Can you work these out from the model? Positions are in its coordinate system, mm. A direction names the side the tool comes from. Give positions to 0.01 mm unless a question says otherwise; leave off trailing zeros. Order: outer loops, then holes, each group sorted by start corner. A loop starts at its lowest first (then second) coordinate and runs counter-clockwise, first axis right, second up. Notation, with made-up numbers: M 44,-14 L 57,-14 A20 ccw 57,3 Z; hole C -36,-2 d3. An arc over 180 degrees is marked long. Write each question's results on one line, items separated by ' | '.
from build123d import *

# Parameters (mm, degrees)
BOSS_EXTRUDE1_DEPTH  = 3.6
CUT_EXTRUDE1_START   = 3.6
CUT_EXTRUDE1_DEPTH   = 1.6
SKETCH3_R            = 0.3
CUT_EXTRUDE2_DEPTH   = 78.737828629
BOSS_EXTRUDE3_DEPTH  = 3
BOSS_EXTRUDE3_TAPER  = 10
SKETCH3_2_R          = 0.3
CUT_EXTRUDE3_DEPTH   = 78.872780874
LPATTERN5_COUNT      = 7
LPATTERN5_PITCH      = 1.27
CHAMFER2_SIZE        = 0.2
FILLET2_R            = 1
BOSS_EXTRUDE4_DEPTH  = 26.2
SKETCH7_R            = 1.05
CUT_EXTRUDE4_DEPTH   = 82.036781772
SKETCH8_W            = 4
SKETCH8_H            = 5.4
CUT_EXTRUDE5_DEPTH   = 1.6
SKETCH9_R            = 1
CUT_EXTRUDE7_DEPTH   = 1
LPATTERN6_COUNT      = 5
LPATTERN6_PITCH      = 2.54
LPATTERN6_COUNT_DIR2 = 2
LPATTERN6_PITCH_DIR2 = 2.54
SKETCH10_R           = 1
CUT_EXTRUDE8_DEPTH   = 1
BOSS_EXTRUDE5_DEPTH  = 1
LPATTERN7_COUNT      = 3
LPATTERN7_PITCH      = 28.5
MIRROR1_COPY_1_DEPTH = 1
MIRROR1_COPY_2_DEPTH = 1
BOSS_EXTRUDE6_DEPTH  = 1
SKETCH14_W           = 6.4
SKETCH14_H           = 0.5
CUT_EXTRUDE9_DEPTH   = 1.55
FILLET3_R            = 1
SKETCH15_R           = 2.794
CUT_EXTRUDE10_DEPTH  = 0.25


with BuildPart() as part:
    # Sketch2 → Boss-Extrude1 (new body)
    with BuildSketch(Plane(origin=(0, 0, 0), x_dir=(1, 0, 0), z_dir=(0, 1, 0))):
        Polygon((0, -2), (-13.1, -2), (-13.1, 68.428427125), (-4.928427125, 76.6), (0, 76.6), (4.928427125, 76.6), (13.1, 68.428427125), (13.1, -2), align=None)
    extrude(amount=BOSS_EXTRUDE1_DEPTH)

    # Sketch1 → Cut-Extrude1 (cut)
    with BuildSketch(Plane(origin=(0, 0, 0), x_dir=(1, 0, 0), z_dir=(0, 1, 0)).offset(CUT_EXTRUDE1_START)):
        Polygon((0, 0), (-11.1, 0), (-11.1, 67.6), (-4.1, 74.6), (0, 74.6), (4.1, 74.6), (11.1, 67.6), (11.1, 0), align=None)
    extrude(amount=-CUT_EXTRUDE1_DEPTH, mode=Mode.SUBTRACT)

    # Sketch3 → Cut-Extrude2 (cut, through all)
    with BuildSketch(Plane(origin=(0, 2, 0), x_dir=(1, 0, 0), z_dir=(0, 1, 0))):
        with Locations(Location((-3.81, 73.66, 0), (0, 0, 270))):
            Circle(SKETCH3_R)
    extrude(amount=-CUT_EXTRUDE2_DEPTH, mode=Mode.SUBTRACT)

    # Sketch5 → Boss-Extrude3 (add)
    with BuildSketch(Plane(origin=(0, 0, 0), x_dir=(-1, 0, 0), z_dir=(0, -1, 0))):
        with BuildLine():
            ThreePointArc((3.81, 72.41), (5.06, 73.66), (3.81, 74.91))
            Line((3.81, 74.91), (-3.782252271, 74.91))
            ThreePointArc((-3.782252271, 74.91), (-5.032252271, 73.66), (-3.782252271, 72.41))
            Line((-3.782252271, 72.41), (3.81, 72.41))
        make_face()
    extrude(amount=BOSS_EXTRUDE3_DEPTH, taper=BOSS_EXTRUDE3_TAPER)

    # Sketch3<2> → Cut-Extrude3 (cut, through all)
    with BuildSketch(Plane(origin=(0, 2, 0), x_dir=(1, 0, 0), z_dir=(0, 1, 0))):
        with Locations(Location((-3.81, 73.66, 0), (0, 0, 270))):
            Circle(SKETCH3_2_R)
    cut_extrude3 = extrude(amount=-CUT_EXTRUDE3_DEPTH, mode=Mode.SUBTRACT)

    # LPattern5: Cut-Extrude3 ×7
    with Locations(*[(i * LPATTERN5_PITCH, 0, 0) for i in range(1, LPATTERN5_COUNT)]):
        add(cut_extrude3, mode=Mode.SUBTRACT)

    # Chamfer2
    chamfer2_edges = [part.edges().sort_by_distance(p)[0] for p in [
        (-3.81, 2, -73.96),
        (-2.54, 2, -73.96),
        (-1.27, 2, -73.96),
        (0, 2, -73.96),
        (1.27, 2, -73.96),
        (2.54, 2, -73.96),
        (3.81, 2, -73.96),
    ]]
    chamfer(chamfer2_edges, length=CHAMFER2_SIZE)

    # Fillet2
    fillet2_edges = [part.edges().sort_by_distance(p)[0] for p in [
        (-5.06, 0, -73.66),
        (-0.013873865, 0, -74.91),
        (5.032252271, 0, -73.66),
        (-0.013873865, 0, -72.41),
    ]]
    fillet(fillet2_edges, radius=FILLET2_R)

    # Sketch6 → Boss-Extrude4 (add)
    with BuildSketch(Plane.ZY.offset(13.1)):
        with BuildLine():
            Line((2, -1), (2, 0))
            Line((2, 0), (-2, 0))
            Line((-2, 0), (-2, -1))
            ThreePointArc((-2, -1), (0, -3), (2, -1))
        make_face()
    extrude(amount=-BOSS_EXTRUDE4_DEPTH)

    # Sketch7 → Cut-Extrude4 (cut, through all)
    with BuildSketch(Plane.ZY.offset(13.1)):
        with Locations((0, -1)):
            Circle(SKETCH7_R)
    extrude(amount=-CUT_EXTRUDE4_DEPTH, mode=Mode.SUBTRACT)

    # Sketch8 → Cut-Extrude5 (cut)
    with BuildSketch(Plane(origin=(0, 3.6, 0), x_dir=(1, 0, 0), z_dir=(0, 1, 0))):
        with Locations((-11.1, 58.5)):
            Rectangle(SKETCH8_W, SKETCH8_H)
    extrude(amount=-CUT_EXTRUDE5_DEPTH, mode=Mode.SUBTRACT)

    # Sketch9 → Cut-Extrude7 (cut)
    with BuildSketch(Plane(origin=(0, 2, 0), x_dir=(1, 0, 0), z_dir=(0, 1, 0))):
        with Locations(Location((-5.08, 4.48, 0), (0, 0, 270))):
            Circle(SKETCH9_R)
    cut_extrude7 = extrude(amount=-CUT_EXTRUDE7_DEPTH, mode=Mode.SUBTRACT)

    # LPattern6: Cut-Extrude7 5 × 2
    with Locations(*[(i * LPATTERN6_PITCH, 0, -j * LPATTERN6_PITCH_DIR2) for i in range(LPATTERN6_COUNT) for j in range(LPATTERN6_COUNT_DIR2) if (i, j) != (0, 0)]):
        add(cut_extrude7, mode=Mode.SUBTRACT)

    # Sketch10 → Cut-Extrude8 (cut)
    with BuildSketch(Plane(origin=(0, 2, 0), x_dir=(1, 0, 0), z_dir=(0, 1, 0))):
        with Locations(Location((0.05, 13.2, 0), (0, 0, 270))):
            Circle(SKETCH10_R)
        with Locations(Location((4.5, 16.25, 0), (0, 0, 270))):
            Circle(SKETCH10_R)
        with Locations(Location((8.95, 13.2, 0), (0, 0, 270))):
            Circle(SKETCH10_R)
        with Locations(Location((8.95, 65.782, 0), (0, 0, 90))):
            Circle(SKETCH10_R)
        with Locations(Location((4.5, 62.732, 0), (0, 0, 90))):
            Circle(SKETCH10_R)
        with Locations(Location((0.05, 65.782, 0), (0, 0, 90))):
            Circle(SKETCH10_R)
    extrude(amount=-CUT_EXTRUDE8_DEPTH, mode=Mode.SUBTRACT)

    # Sketch11 → Boss-Extrude5 (add, symmetric)
    with BuildSketch(Plane.XY.offset(-7)):
        Polygon((-11.1, 3.6), (-11.1, 5.6), (-11.75, 5.6), (-12.18, 4.855218153), (-12.18, 4.720110177), (-11.85, 4.6), (-11.85, 3.6), align=None)
    boss_extrude5 = extrude(amount=BOSS_EXTRUDE5_DEPTH, both=True)

    # LPattern7: Boss-Extrude5 ×3
    with Locations(*[(0, 0, -i * LPATTERN7_PITCH) for i in range(1, LPATTERN7_COUNT)]):
        add(boss_extrude5)

    # Mirror1: Boss-Extrude5 across plane
    add(boss_extrude5.mirror(Plane(origin=(0, 0, 0), x_dir=(0, 0, 1), z_dir=(1, 0, 0))))

    # Mirror1 copy 1 sketch → Mirror1 copy 1 (add, symmetric)
    with BuildSketch(Plane(origin=(0, 0, -35.5), x_dir=(-1, 0, 0), z_dir=(0, 0, 1))):
        Polygon((-11.1, -3.6), (-11.1, -5.6), (-11.75, -5.6), (-12.18, -4.855218153), (-12.18, -4.720110177), (-11.85, -4.6), (-11.85, -3.6), align=None)
    extrude(amount=MIRROR1_COPY_1_DEPTH, both=True)

    # Mirror1 copy 2 sketch → Mirror1 copy 2 (add, symmetric)
    with BuildSketch(Plane(origin=(0, 0, -64), x_dir=(-1, 0, 0), z_dir=(0, 0, 1))):
        Polygon((-11.1, -3.6), (-11.1, -5.6), (-11.75, -5.6), (-12.18, -4.855218153), (-12.18, -4.720110177), (-11.85, -4.6), (-11.85, -3.6), align=None)
    extrude(amount=MIRROR1_COPY_2_DEPTH, both=True)

    # Sketch13 → Boss-Extrude6 (add, symmetric)
    with BuildSketch(Plane(origin=(0, 0, 0), x_dir=(0, 0, -1), z_dir=(1, 0, 0))):
        Polygon((0, 3.6), (0, 5.6), (-0.65, 5.6), (-1.08, 4.855218153), (-1.08, 4.720110177), (-0.75, 4.6), (-0.75, 3.6), align=None)
    boss_extrude6 = extrude(amount=BOSS_EXTRUDE6_DEPTH, both=True)

    # Mirror2: Boss-Extrude6 across plane
    add(boss_extrude6.mirror(Plane.XY.offset(-37.3)))

    # Sketch14 → Cut-Extrude9 (cut)
    with BuildSketch(Plane(origin=(-11.1, 0, 0), x_dir=(0, 0, -1), z_dir=(1, 0, 0))):
        with Locations((58.5, 2.95)):
            Rectangle(SKETCH14_W, SKETCH14_H)
    extrude(amount=-CUT_EXTRUDE9_DEPTH, mode=Mode.SUBTRACT)

    # Fillet3
    fillet3_edges = [part.edges().sort_by_distance(p)[0] for p in [
        (0, 0, -2),
    ]]
    fillet(fillet3_edges, radius=FILLET3_R - 0.0001)  # a hair under: the kernel refuses the full size

    # Sketch15 → Cut-Extrude10 (cut)
    with BuildSketch(Plane.XZ):
        with Locations(Location((0, -10, 0), (0, 0, 270))):
            Circle(SKETCH15_R)
    extrude(amount=-CUT_EXTRUDE10_DEPTH, mode=Mode.SUBTRACT)


solid = part.part
(1) For faces 4 (the face through (-0.183, -1.932, 0.485)), 5 (the face through (-12.1, 2.5, -61.2)), 6 (the face through (2.84, 1.507, -3.526)), which set-ups out of +Z, -Z, +X, -X, +Y, -Y let a thin tool reach every point of the face, with its end or its side?
Data:
face 4: +X, -X | face 5: -X, +Y | face 6: +Y
(2) I need wall thicknesses on L1, parallel to X at y = 1.75, z = -4.48; L2, parallel to X at y = 1.45, z = -13.2; L3, parallel to X at y = 3.25, z = -5.5. Which ranges of each line are inside material? Lowest first, please. Write a range as from..to.
Data:
L1: x = -13.1..-6.08, -4.08..-3.54, -1.54..-1, 1..1.54, 3.54..4.08, 6.08..13.1 | L2: x = -13.1..-0.95, 1.05..7.95, 9.95..13.1 | L3: x = -13.1..-11.1, 11.1..13.1
(3) Imagine slicing it at C-C, the plane z = -59. Write out the boundary of the cut face in (x, y).
Data:
outline: M -13.1,0 L 13.1,0 L 13.1,3.6 L 11.1,3.6 L 11.1,2 L -13.1,2 Z
(4) Imagine slicing it at A-A, the plane z = -48. Write out the boundary of the cut face in (x, y), plus the area to 3 significant figures.
Data:
outline: M -13.1,0 L 13.1,0 L 13.1,3.6 L 11.1,3.6 L 11.1,2 L -11.1,2 L -11.1,3.6 L -13.1,3.6 Z | area: 58.8 mm2
(5) Will these pins go through, and if not, where does the flat tip stop? P1, Ø4, axis at x = 3.5, z = -25.5, coming from the -Y side; P2, Ø1, axis at x = -0.5, z = -13.5, coming from the +Y side; P3, Ø1.5, axis at x = -5, y = 1, coming from the -Z side; P4, Ø1.8, axis at x = 8.95, z = -65.782, coming from the +Y side.
Data:
P1: stops at y = 0 | P2: stops at y = 2 | P3: stops at z = -76.6 | P4: stops at y = 1
(6) We'd pull the mould along Z, two halves only. Please class faces 1 (the face through (13.1, 2, -34)), 2 (the face through (0, 2, -76.6)), 3 (the face through (0, 0.25, -10)): +Z half, -Z half, draft (parallel to the pull), parting line (faces both ways), or undercut.
Data:
face 1: draft | face 2: -Z half | face 3: undercut
